Geometry check sheet. Reference: the model listing, model coordinates, mm. Face numbers are marked on the shaded views. A direction names the side the tool comes from. Coordinates: 2 decimals unless noted, no trailing zeros. Loops run counter-clockwise (first coordinate to the right, second up) from the corner with the lowest first, then second, coordinate; pieces in that order, holes last.
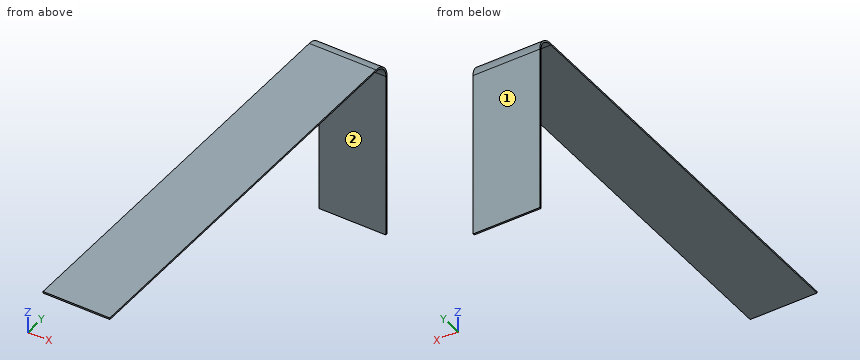
Autodesk Inventor part; units mm, degrees
ref_plane "YZ Plane" through (0, 0, 0) normal (1, 0, 0) x (0, 1, 0)
ref_plane "XZ Plane" through (0, 0, 0) normal (0, 1, 0) x (-1, 0, 0)
ref_plane "XY Plane" through (0, 0, 0) normal (0, 0, 1) x (1, 0, 0)
sketch "Sketch1" plane through (0, 0, 0) normal (0, 1, 0) x (-1, 0, 0)
  line L0 (-2, 18) -> (-2, -18)
  line L1 (-2, -18) -> (2, -18)
  line L2 (2, -18) -> (2, 18)
  line L3 (2, 18) -> (-2, 18)
  line L4 (-2, 18) -> (2, -18) construction
  line L5 (-2, -18) -> (2, 18) construction
  point P0 (0, 0)
extrude "Extrusion1" add sketch "Sketch1" along normal blind 0.1
sketch "Sketch2" plane through (0, 0.1, 0) normal (0, 1, 0) x (1, 0, 0)
  line L0 (2, -18) -> (2, 18)
  line L1 (2, 18) -> (-2, 18)
  line L2 (-2, 18) -> (-2, -18)
  line L3 (-2, 8) -> (2, 8)
  point P0 (0, 0)
  dimension "d2" = 10
bend part "Bend Part1" radius 1 angle 90 line through (-2, 0.1, -8) along (1, 0, 0) centre toward (0, -1, 0) moving side (0, 0, 1) both sides no
properties part number "PIElectrodes"
1) Section check B-B on z = -12.25. Record the cut outline in (x, y).
Data:
outline: (-2, 0) - (2, 0) - (2, 0.1) - (-2, 0.1) - close
2) Section check C-C on y = -3.5. Record the cut outline in (x, z), and give its area (3 significant figures).
Data:
outline: (-2, -7.1) - (2, -7.1) - (2, -7) - (-2, -7) - close
area: 0.400 mm2
3) Access from +Z, -Z, +X, -X, +Y, -Y to the whole of each face (thin tool, end or side, straight path). Record for the marked faces 1 and 2.
Data:
face 1: +Z, -Z, +X, -X, +Y
face 2: -Z, +X, -X, -Y
4) Section check A-A on x = -1.55. Record the cut outline in (y, z), and give its area (3 significant figures).
Data:
outline: (-25.33, -7.1) - (-0.9, -7.1) arc R0.9 cw to (0, -8) - (0, -18) - (0.1, -18) - (0.1, -8) arc R1 ccw to (-0.9, -7) - (-25.33, -7) - close
area: 3.59 mm2
